Work out the finished part from the listing and answer in its coordinate system (mm). A direction names the side the tool comes from. Give positions to 0.01 mm unless a question says otherwise; leave off trailing zeros. Loops run counter-clockwise (first coordinate to the right, second up) from the corner with the lowest first, then second, coordinate; pieces in that order, holes last. Notation, with made-up numbers: (16.25, -15.5) - (39.25, -15.5) arc R16 ccw to (39.25, 5.5) - close; hole circle Ø9 at (29.25, 24). An arc over 180 degrees is marked (long way). One line per question, with ' | ' between items. Start each with the question number.
1. Section B-B (z = 5.25) is taken. Determine the outline of the cut face in (x, y), plus the area to 3 significant figures.
2. Section A-A (x = 0) is taken. Determine the outline of the cut face in (y, z), plus the area to 3 significant figures.
3. For a pull along Y with two mould halves and no side action, classify faces 6 (the face through (-48, 12.698, 3)), 7 (the face through (44.45, 3, 3)), 8 (the face through (-48, 33.652, 3)) as released by +Y, released by -Y, zero draft, split by the parting line, or undercut.
4. Each of these flat-tipped pins is pushed along its axis until it touches: pin 1 (3 mm diameter, centred on y = 19.5, z = 2, fed in from -X); pin 2 (3 mm diameter, centred on x = -6.5, z = 2, fed in from -Y); pin 3 (3 mm diameter, centred on y = 2.5, z = 3, fed in from +X); pin 4 (3 mm diameter, centred on x = -48, z = 4, fed in from -Y). Where does it stop, or does it pass through?
5. Which of the six approach directions +Z, -Z, +X, -X, +Y, -Y give full straight-line access (tool end or side, diameter ignored) to faces 1 (the face through (48, 12.698, 3)), 2 (the face through (-44.45, 3, 3)), 3 (the face through (44.45, 37, 3)), 4 (the face through (-44.45, 37, 3)), 5 (the face through (48, 6.348, 3))?
6. Find the intervals of material crossed by line 1 (Y direction, x = 0, z = 2.75); line 2 (X direction, y = 34, z = 3.75); line 3 (X direction, y = 22, z = 5.25), in increasing order.
7. Section D-D (y = 37.5) is taken. Determine the outline of the cut face in (x, z).
8. Section C-C (y = 17.5) is taken. Determine the outline of the cut face in (x, z).
Autodesk Inventor part; units mm, degrees
ref_plane "YZ Plane" through (0, 0, 0) normal (1, 0, 0) x (0, 1, 0)
ref_plane "XZ Plane" through (0, 0, 0) normal (0, 1, 0) x (-1, 0, 0)
ref_plane "XY Plane" through (0, 0, 0) normal (0, 0, 1) x (1, 0, 0)
sketch "Sketch1" plane through (0, 0, 0) normal (0, 0, 1) x (1, 0, 0)
  line L0 (-44.45, 0) -> (44.45, 0)
  line L1 (44.45, 0) -> (44.45, 40)
  line L2 (44.45, 40) -> (-44.45, 40)
  line L3 (-44.45, 40) -> (-44.45, 0)
  line L4 (-50.8, 33.6525) -> (-44.45, 33.6525)
  line L5 (-44.45, 33.6525) -> (-44.45, 27.3025)
  line L6 (-44.45, 27.3025) -> (-50.8, 27.3025)
  line L7 (-50.8, 27.3025) -> (-50.8, 33.6525)
  line L8 (-50.8, 12.6975) -> (-44.45, 12.6975)
  line L9 (-44.45, 12.6975) -> (-44.45, 6.3475)
  line L10 (-44.45, 6.3475) -> (-50.8, 6.3475)
  line L11 (-50.8, 6.3475) -> (-50.8, 12.6975)
  line L12 (0, 40) -> (0, 32.8851)
  line L13 (-44.45, 12.6975) -> (-44.45, 27.3025)
  line L14 (50.8, 33.6525) -> (44.45, 33.6525)
  line L15 (44.45, 33.6525) -> (44.45, 27.3025)
  line L16 (44.45, 27.3025) -> (50.8, 27.3025)
  line L17 (50.8, 27.3025) -> (50.8, 33.6525)
  line L18 (50.8, 12.6975) -> (44.45, 12.6975)
  line L19 (44.45, 12.6975) -> (44.45, 6.3475)
  line L20 (44.45, 6.3475) -> (50.8, 6.3475)
  line L21 (50.8, 6.3475) -> (50.8, 12.6975)
  line L22 (44.45, 12.6975) -> (44.45, 27.3025)
  point P0 (0, 0)
  point P1 (-44.45, 20)
  point P2 (0, 0)
  point P3 (44.45, 20)
  dimension "d0" = 40
  dimension "d1" = 88.9
  dimension "d2" = 6.35
  dimension "d3" = 6.35
  dimension "d4" = 14.605
extrude "Extrusion1" add sketch "Sketch1" along normal blind 6.35
hole "Hole1" at (0, 20.0102, 6.35) direction (0, 0, -1) diameter 8.9916 end through all
properties part number "acrylic kinect plate"
Conclusion:
1) outline: (-50.8, 6.35) - (-44.45, 6.35) - (-44.45, 0) - (44.45, 0) - (44.45, 6.35) - (50.8, 6.35) - (50.8, 12.7) - (44.45, 12.7) - (44.45, 27.3) - (50.8, 27.3) - (50.8, 33.65) - (44.45, 33.65) - (44.45, 40) - (-44.45, 40) - (-44.45, 33.65) - (-50.8, 33.65) - (-50.8, 27.3) - (-44.45, 27.3) - (-44.45, 12.7) - (-50.8, 12.7) - close; hole circle Ø8.99 at (0, 20.01) | area: 3,650 mm²
2) outline: (0, 0) - (15.51, 0) - (15.51, 6.35) - (0, 6.35) - close; (24.51, 0) - (40, 0) - (40, 6.35) - (24.51, 6.35) - close | area: 197 mm²
3) face 6: undercut | face 7: zero draft | face 8: released by +Y
4) pin 1: x = -44.45 | pin 2: y = 0 | pin 3: x = 44.45 | pin 4: y = 6.35
5) face 1: +Z, -Z, +X | face 2: +Z, -Z, -X, -Y | face 3: +Z, -Z, +X, +Y | face 4: +Z, -Z, -X, +Y | face 5: +Z, -Z, +X, -Y
6) line 1: 0 to 15.51, 24.51 to 40 | line 2: -44.45 to 44.45 | line 3: -44.45 to -4.03, 4.03 to 44.45
7) outline: (-44.45, 0) - (44.45, 0) - (44.45, 6.35) - (-44.45, 6.35) - close
8) outline: (-44.45, 0) - (-3.73, 0) - (-3.73, 6.35) - (-44.45, 6.35) - close; (3.73, 0) - (44.45, 0) - (44.45, 6.35) - (3.73, 6.35) - close
